```python
from build123d import *

# Parameters (mm, degrees)
SKETCH1_R           = 1.6
BOSS_EXTRUDE1_DEPTH = 3.175
SKETCH2_R           = 1.6
SKETCH2_R_2         = 7.5
CUT_EXTRUDE1_DEPTH  = 4.175
BOSS_EXTRUDE3_DEPTH = 3.175


with BuildPart() as part:
    # Sketch1 → Boss-Extrude1 (new body)
    with BuildSketch(Plane.XY):
        with BuildLine():
            Line((31.086717458, 32.79124845), (24.539210672, 37.049362302))
            ThreePointArc((24.539210672, 37.049362302), (22.268882249, 37.695107847), (20.029743315, 36.948358029))
            Line((20.029743315, 36.948358029), (13.602836128, 32.346493758))
            ThreePointArc((13.602836128, 32.346493758), (12.968237383, 31.781029757), (12.467444066, 31.094246563))
            Line((12.467444066, 31.094246563), (1.349560594, 11.837507517))
            ThreePointArc((1.349560594, 11.837507517), (0.995156132, 11.028730142), (0.826837821, 10.16190126))
            Line((0.826837821, 10.16190126), (0.217529035, 2.673448792))
            ThreePointArc((0.217529035, 2.673448792), (0.712425098, 0.398045931), (2.390731369, -1.216162343))
            Line((2.390731369, -1.216162343), (9.39530455, -4.779380795))
            ThreePointArc((9.39530455, -4.779380795), (10.276421795, -5.10394936), (11.208926603, -5.214163404))
            Line((11.208926603, -5.214163404), (33.291073397, -5.214163404))
            ThreePointArc((33.291073397, -5.214163404), (34.223578205, -5.10394936), (35.10469545, -4.779380795))
            Line((35.10469545, -4.779380795), (42.181392008, -1.179473262))
            ThreePointArc((42.181392008, -1.179473262), (43.83187157, 0.385744129), (44.362149812, 2.597710054))
            Line((44.362149812, 2.597710054), (43.941412908, 10.526262814))
            ThreePointArc((43.941412908, 10.526262814), (43.781938908, 11.451617014), (43.411134666, 12.314296889))
            Line((43.411134666, 12.314296889), (32.370061269, 31.437996983))
            ThreePointArc((32.370061269, 31.437996983), (31.808360702, 32.190462814), (31.086717458, 32.79124845))
        make_face()
        with Locations((13.589745962, 17.846043489)):
            Circle(SKETCH1_R, mode=Mode.SUBTRACT)
        with Locations((9.526279442, 5.5)):
            Circle(SKETCH1_R, mode=Mode.SUBTRACT)
        with Locations((34.973720558, 5.5)):
            Circle(SKETCH1_R, mode=Mode.SUBTRACT)
        with Locations((30.910254038, 17.846043489)):
            Circle(SKETCH1_R, mode=Mode.SUBTRACT)
        with Locations((22.25, 27.538130468)):
            Circle(SKETCH1_R, mode=Mode.SUBTRACT)
        with Locations((22.25, 2.846043489)):
            Circle(SKETCH1_R, mode=Mode.SUBTRACT)
        with BuildLine():
            Line((42.370834875, 9.312177826), (35.370834875, -2.812177826))
            ThreePointArc((35.370834875, -2.812177826), (34.687822174, -2.995190528), (34.504809472, -2.312177826))
            Line((34.504809472, -2.312177826), (41.504809472, 9.812177826))
            ThreePointArc((41.504809472, 9.812177826), (42.187822174, 9.995190528), (42.370834875, 9.312177826))
        make_face(mode=Mode.SUBTRACT)
        with BuildLine():
            Line((10.01754221, -2.349929674), (3.01754221, 9.774425979))
            ThreePointArc((3.01754221, 9.774425979), (2.334529508, 9.957438681), (2.151516806, 9.274425979))
            Line((2.151516806, 9.274425979), (9.151516806, -2.849929674))
            ThreePointArc((9.151516806, -2.849929674), (9.834529508, -3.032942376), (10.01754221, -2.349929674))
        make_face(mode=Mode.SUBTRACT)
        with BuildLine():
            Line((15.358452868, 31.038130468), (29.358452868, 31.038130468))
            ThreePointArc((29.358452868, 31.038130468), (29.858452868, 31.538130468), (29.358452868, 32.038130468))
            Line((29.358452868, 32.038130468), (15.358452868, 32.038130468))
            ThreePointArc((15.358452868, 32.038130468), (14.858452868, 31.538130468), (15.358452868, 31.038130468))
        make_face(mode=Mode.SUBTRACT)
    extrude(amount=BOSS_EXTRUDE1_DEPTH)

    # Sketch2 → Cut-Extrude1 (cut, through all)
    with BuildSketch(Plane.XY.offset(3.175)):
        with Locations((41.761034996, 1.563830145)):
            Circle(SKETCH2_R)
        with Locations((2.789891826, 1.563830145)):
            Circle(SKETCH2_R)
        with Locations((22.275463411, 12.813830145)):
            Circle(SKETCH2_R_2)
        with Locations((22.275463411, 35.313830145)):
            Circle(SKETCH2_R)
    extrude(amount=-CUT_EXTRUDE1_DEPTH, mode=Mode.SUBTRACT)

    # Sketch3 → Boss-Extrude3 (add)
    with BuildSketch(Plane.XY.offset(3.175)):
        with BuildLine():
            Line((42.370834875, 9.312177826), (35.370834875, -2.812177826))
            ThreePointArc((35.370834875, -2.812177826), (34.687822174, -2.995190528), (34.504809472, -2.312177826))
            Line((34.504809472, -2.312177826), (41.504809472, 9.812177826))
            ThreePointArc((41.504809472, 9.812177826), (42.187822174, 9.995190528), (42.370834875, 9.312177826))
        make_face()
        with BuildLine():
            Line((10.01754221, -2.349929674), (3.01754221, 9.774425979))
            ThreePointArc((3.01754221, 9.774425979), (2.334529508, 9.957438681), (2.151516806, 9.274425979))
            Line((2.151516806, 9.274425979), (9.151516806, -2.849929674))
            ThreePointArc((9.151516806, -2.849929674), (9.834529508, -3.032942376), (10.01754221, -2.349929674))
        make_face()
        with BuildLine():
            Line((15.358452868, 31.038130468), (29.358452868, 31.038130468))
            ThreePointArc((29.358452868, 31.038130468), (29.858452868, 31.538130468), (29.358452868, 32.038130468))
            Line((29.358452868, 32.038130468), (15.358452868, 32.038130468))
            ThreePointArc((15.358452868, 32.038130468), (14.858452868, 31.538130468), (15.358452868, 31.038130468))
        make_face()
    extrude(amount=-BOSS_EXTRUDE3_DEPTH)


solid = part.part
```
Geometry: final body of the model. Coordinates: model frame, mm. Round coordinates to 2 decimals unless told otherwise and drop trailing zeros. Loops run counter-clockwise (first coordinate to the right, second up) from the corner with the lowest first, then second, coordinate; pieces in that order, holes last. Notation, with made-up numbers: (6, -36.75) -> (24, -36.75) arc R22 cw to (24, -5.75) -> close; hole circle Ø1 at (-10.75, 64.25). An arc over 180 degrees is marked (long way). Use one line per item in the form item = value.
Item 1: Cut plane C-C on x = 22.25. Output: boundary loops of the cut face in (y, z) (3 decimals), then the cut area to 3 significant figures.
Evaluation:
outline = (-5.214, 0) -> (1.246, 0) -> (1.246, 3.175) -> (-5.214, 3.175) -> close; (4.446, 0) -> (5.314, 0) -> (5.314, 3.175) -> (4.446, 3.175) -> close; (20.314, 0) -> (25.938, 0) -> (25.938, 3.175) -> (20.314, 3.175) -> close; (29.138, 0) -> (33.714, 0) -> (33.714, 3.175) -> (29.138, 3.175) -> close; (36.914, 0) -> (37.695, 0) -> (37.695, 3.175) -> (36.914, 3.175) -> close
area = 58.1 mm2
Item 2: Contact query for flat-ended pins moving along their axis: pin 1 Ø3 at (x, y) = (9.53, 5.5) entering from +Z; pin 2 Ø1 at (y, z) = (26.5, 0.5) entering from +X. Output: stop coordinate, or through.
Evaluation:
pin_1 = through
pin_2 = 35.51
Item 3: Cut plane B-B on z = 1.5. Give the number of separate pieces and of enclosed holes in the cut face, then the cut area to 3 significant figures.
Evaluation:
separate_pieces = 1
enclosed_holes = 10
area = 1,120 mm2
Item 4: Cut plane A-A on y = 9. Output: boundary loops of the cut face in (x, z) (3 decimals), then the cut area to 3 significant figures.
Evaluation:
outline = (0.732, 0) -> (15.818, 0) -> (15.818, 3.175) -> (0.732, 3.175) -> close; (28.733, 0) -> (44.022, 0) -> (44.022, 3.175) -> (28.733, 3.175) -> close
area = 96.4 mm2
Item 5: Cut plane D-D on y = 34.5. Output: boundary loops of the cut face in (x, z) (3 decimals), then the cut area to 3 significant figures.
Evaluation:
outline = (16.61, 0) -> (20.898, 0) -> (20.898, 3.175) -> (16.61, 3.175) -> close; (23.653, 0) -> (28.459, 0) -> (28.459, 3.175) -> (23.653, 3.175) -> close
area = 28.9 mm2
Item 6: Material intervals for probe 1 along Y at (x, z) = (22.25, 0.8); probe 2 along X at (y, z) = (2, 3); probe 3 along X at (y, z) = (6, 0.4), sorted ascending.
Evaluation:
probe_1 = -5.21 to 1.25, 4.45 to 5.31, 20.31 to 25.94, 29.14 to 33.71, 36.91 to 37.69
probe_2 = 0.22 to 1.25, 4.33 to 20.89, 23.61 to 40.22, 43.3 to 44.35
probe_3 = 0.49 to 8.01, 11.05 to 19.14, 25.41 to 33.45, 36.49 to 44.18
Item 7: Draft query along Y for faces 1 (the cylindrical face through (31.8, 32.2, 1.6)), 2 (the flat face through (17, 7, 0)), 3 (the cylindrical face through (22.99, 26.12, 1.57)). Return one class per face: released by +Y, released by -Y, zero draft, split by the parting line, or undercut.
Evaluation:
face_1 = released by +Y
face_2 = zero draft
face_3 = undercut
